from build123d import *

# Parameters (mm, degrees)
F0_W     = 25.4
F0_H     = 93.98
F1_DEPTH = 3.048
F2_SIZE2 = 91.44
F2_SIZE  = 22.86
F3_SIZE2 = 6.35
F3_SIZE  = 6.35


with BuildPart() as f1:
    # F0 (on Front) → F1 (new body)
    with BuildSketch(Plane.XZ):
        Rectangle(F0_W, F0_H)
    extrude(amount=F1_DEPTH)

    # F2
    f2_edges = [f1.edges().sort_by_distance(p)[0] for p in [
        (-12.7, -1.524, 46.99),
    ]]
    f2_side = f1.faces().sort_by_distance((0, -1.524, 46.99))[0]
    chamfer(f2_edges, length=F2_SIZE, length2=F2_SIZE2, reference=f2_side)

    # F3
    f3_edges = [f1.edges().sort_by_distance(p)[0] for p in [
        (12.7, -1.524, -46.99),
    ]]
    chamfer(f3_edges, length=F3_SIZE, length2=F3_SIZE2)


solid = f1.part
Could you check a few things on this model? Use its own coordinates, in mm. Give positions to 0.01 mm unless a question says otherwise; leave off trailing zeros. Order: outer loops, then holes, each group sorted by start corner. A loop starts at its lowest first (then second) coordinate and runs counter-clockwise, first axis right, second up.
Item 1: If we section it at C-C, the plane z = 15.5: Write out the boundary of the cut face in (x, y), plus the area to 3 significant figures.
Item 2: If we section it at B-B, the plane y = -0.7: Write out the boundary of the cut face in (x, z), plus the area to 3 significant figures.
Item 3: I need wall thicknesses on line 1 (X direction, y = -2.65, z = 39.5); line 2 (X direction, y = -1.7, z = 43). Which ranges of each line are inside material? Lowest first, please.
Item 4: If we section it at A-A, the plane x = 7.25: Write out the boundary of the cut face in (y, z).
Values:
1. outline: (2.29, -3.05) - (12.7, -3.05) - (12.7, 0) - (2.29, 0) - close
1. area: 31.7 mm2
2. outline: (-12.7, -46.99) - (6.35, -46.99) - (12.7, -40.64) - (12.7, 46.99) - (10.16, 46.99) - (-12.7, -44.45) - close
2. area: 1,320 mm2
3. line 1: x = 8.29 to 12.7
3. line 2: x = 9.16 to 12.7
4. outline: (-3.05, -46.09) - (0, -46.09) - (0, 35.35) - (-3.05, 35.35) - close
